The model under review builds one solid part; all positions refer to its coordinate system, in mm. Coordinates: 2 decimals unless noted, no trailing zeros. Loops run counter-clockwise (first coordinate to the right, second up) from the corner with the lowest first, then second, coordinate; pieces in that order, holes last. Notation, with made-up numbers: (21, 44) - (44, 44) arc R21 cw to (44, 61) - close; hole circle Ø2 at (73.5, -34). An arc over 180 degrees is marked (long way). One line per item, written item: value. Start each with the question number.
1. We need section D-D, the plane x = 0. Give the boundary of the cut face in (y, z).
2. Mouldability with a two-part tool opening along Z and no side actions: class faces 1 (the face through (30.162, 0, 0)), 2 (the face through (19.45, -0.09, 1.26)), 3 (the face through (0, -1, 6.35)) as +Z half, -Z half, draft (parallel to the pull), parting line (faces both ways), or undercut.
3. We need section B-B, the plane x = -22.5. Give the boundary of the cut face in (y, z), then the cut area to 4 significant figures.
4. We need section C-C, the plane y = -0.25. Give the boundary of the cut face in (x, z), then the cut area to 3 significant figures.
5. To check wall thickness, follow line 1 (X direction, y = 5.5, z = 0.25); line 2 (Z direction, x = -22.5, y = 2.5); line 3 (X direction, y = 0.25, z = 3). State the ranges of each line that lie inside material, in increasing order.
6. We need section A-A, the plane z = 0. Give the boundary of the cut face in (x, y), then the cut area to 3 significant figures.
from build123d import *

# Parameters (mm, degrees)
SKETCH1_W            = 12.7
SKETCH1_H            = 12.7
BOSS_EXTRUDE1_DEPTH  = 30.1625
M6_CLEARANCE_HOLE1_D = 6.6
CHAMFER1_SIZE        = 1.5875


with BuildPart() as part:
    # Sketch1 → Boss-Extrude1 (new, symmetric)
    with BuildSketch(Plane(origin=(0, 0, 0), x_dir=(0, 0, -1), z_dir=(1, 0, 0))):
        Rectangle(SKETCH1_W, SKETCH1_H)
    extrude(amount=BOSS_EXTRUDE1_DEPTH, both=True)

    # M6 Clearance Hole1 (through all)
    with Locations(Plane(origin=(0, 6.35, 0), x_dir=(1, 0, 0), z_dir=(0, 1, 0))):
        with Locations((-22.5, 0), (22.5, 0)):
            Hole(M6_CLEARANCE_HOLE1_D / 2)

    # Chamfer1
    chamfer1_edges = [part.edges().sort_by_distance(p)[0] for p in [
        (0, 6.35, 6.35),
        (0, 6.35, -6.35),
    ]]
    chamfer(chamfer1_edges, length=CHAMFER1_SIZE)


solid = part.part
Findings below:
1. outline: (-6.35, -6.35) - (4.76, -6.35) - (6.35, -4.76) - (6.35, 4.76) - (4.76, 6.35) - (-6.35, 6.35) - close
2. face 1: draft
2. face 2: undercut
2. face 3: +Z half
3. outline: (-6.35, -6.35) - (4.76, -6.35) - (6.35, -4.76) - (6.35, -3.3) - (-6.35, -3.3) - close; (-6.35, 3.3) - (6.35, 3.3) - (6.35, 4.76) - (4.76, 6.35) - (-6.35, 6.35) - close
3. area: 74.95 mm2
4. outline: (-30.16, -6.35) - (30.16, -6.35) - (30.16, 6.35) - (-30.16, 6.35) - close; hole circle Ø6.6 at (-22.5, 0); hole circle Ø6.6 at (22.5, 0)
4. area: 698 mm2
5. line 1: -30.16 to -25.79, -19.21 to 19.21, 25.79 to 30.16
5. line 2: -6.35 to -3.3, 3.3 to 6.35
5. line 3: -30.16 to -23.87, -21.13 to 21.13, 23.87 to 30.16
6. outline: (-30.16, -6.35) - (-25.8, -6.35) - (-25.8, 6.35) - (-30.16, 6.35) - close; (-19.2, -6.35) - (19.2, -6.35) - (19.2, 6.35) - (-19.2, 6.35) - close; (25.8, -6.35) - (30.16, -6.35) - (30.16, 6.35) - (25.8, 6.35) - close
6. area: 598 mm2
